Could you check a few things on this model? Use its own coordinates, in mm. Face numbers are marked on the shaded views. A direction names the side the tool comes from. Round coordinates to 2 decimals unless told otherwise and drop trailing zeros. Loops run counter-clockwise (first coordinate to the right, second up) from the corner with the lowest first, then second, coordinate; pieces in that order, holes last. Notation, with made-up numbers: (88, 72.5) - (121, 72.5) arc R13 cw to (121, 93.5) - close; hole circle Ø2 at (-5.75, -5). An arc over 180 degrees is marked (long way). Put each result on its own line as item: value. Start each with the question number.
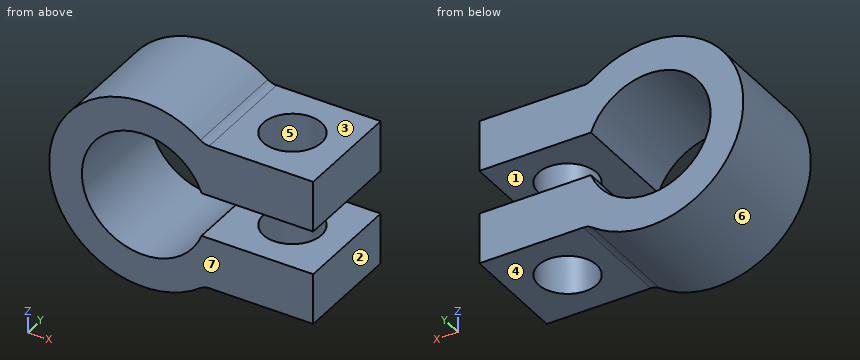
from build123d import *

# Parameters (mm, degrees)
SCHIZZO3_R           = 13
SCHIZZO3_R_2         = 8.5
ANELLO_DEPTH         = 15
AGGANCIOALTO_DEPTH   = 15
SCHIZZO5_W           = 23.306623863
SCHIZZO5_H           = 6
APERTURAANELLO_DEPTH = 31.61370144
SCHIZZO6_R           = 4
FOROPASSANTE_DEPTH   = 37.016644984
RACCORDOBASSO_R      = 2
RACCORDOALTO_R       = 2


with BuildPart() as part:
    # Schizzo3 → Anello (new body)
    with BuildSketch(Plane(origin=(0, 0, 0), x_dir=(1, 0, 0), z_dir=(0, 1, 0))):
        with Locations(Location((0, 0, 0), (0, 0, 270))):
            Circle(SCHIZZO3_R)
        with Locations(Location((0, 0, 0), (0, 0, 270))):
            Circle(SCHIZZO3_R_2, mode=Mode.SUBTRACT)
    extrude(amount=ANELLO_DEPTH)

    # Schizzo4 → AggancioAlto (add)
    with BuildSketch(Plane(origin=(0, 0, 0), x_dir=(1, 0, 0), z_dir=(0, 1, 0))):
        with BuildLine():
            Line((23.306623863, 3), (12.649110641, 3))
            ThreePointArc((12.649110641, 3), (11.046977059, 6.853050259), (8.306623863, 10))
            Line((8.306623863, 10), (23.306623863, 10))
            Line((23.306623863, 10), (23.306623863, 3))
        make_face()
    aggancioalto = extrude(amount=AGGANCIOALTO_DEPTH)

    # AggancioBasso: AggancioAlto across plane
    add(aggancioalto.mirror(Plane.XY))

    # Schizzo5 → AperturaAnello (cut, through all)
    with BuildSketch(Plane(origin=(0, 15, 0), x_dir=(1, 0, 0), z_dir=(0, 1, 0))):
        with Locations((11.653311932, 0)):
            Rectangle(SCHIZZO5_W, SCHIZZO5_H)
    extrude(amount=-APERTURAANELLO_DEPTH, mode=Mode.SUBTRACT)

    # Schizzo6 → ForoPassante (cut, through all)
    with BuildSketch(Plane.XY.offset(10)):
        with Locations((15.806623863, 7.5)):
            Circle(SCHIZZO6_R)
    extrude(amount=-FOROPASSANTE_DEPTH, mode=Mode.SUBTRACT)

    # RaccordoBasso
    raccordobasso_edges = [part.edges().sort_by_distance(p)[0] for p in [
        (8.306623863, 7.5, 10),
    ]]
    fillet(raccordobasso_edges, radius=RACCORDOBASSO_R)

    # RaccordoAlto
    raccordoalto_edges = [part.edges().sort_by_distance(p)[0] for p in [
        (8.306623863, 7.5, -10),
    ]]
    fillet(raccordoalto_edges, radius=RACCORDOALTO_R)


solid = part.part
Item 1: Suppose I cut it at C-C, the plane z = -7.75. List the corners of the cut face in (x, y) for me.
Item 2: Suppose I cut it at D-D, the plane x = 18.5. List the corners of the cut face in (y, z) for me.
Item 3: I need wall thicknesses on line 1 (Z direction, x = 21, y = 2.5); line 2 (Z direction, x = 0, y = 9.75); line 3 (X direction, y = 10, z = -7.75). Which ranges of each line are inside material? Lowest first, please. Write a range as from..to.
Item 4: Will these pins go through, and if not, where does the flat tip stop? P1, Ø3, axis at y = 5, z = 9.5, coming from the -X side; P2, Ø4.5, axis at x = 14.5, y = 9, coming from the +Z side; P3, Ø7.5, axis at x = 18.5, y = 9.5, coming from the -Z side.
Item 5: Suppose I cut it at B-B, the plane x = 0. List the corners of the cut face in (y, z) for me, then the cut area to 3 significant figures.
Item 6: On a 3-axis mill with a long thin cutter (end or side, diameter ignored), from which of +Z, -Z, +X, -X, +Y, -Y can I reach the whole of each face in a straight line? I mean the marked faces 1, 2, 3 and 4. Say none if no direction works.
Item 7: Suppose I cut it at A-A, the plane y = 7.5. List the corners of the cut face in (x, z) for me, then the cut area to 3 significant figures.
Item 8: Thinking about a two-plate mould opening in Y: for the marked faces 5, 6 and 7, which applies, released by +Y, released by -Y, zero draft, split by the parting line, or undercut?
Numbers:
1. outline: (-10.44, 0) - (-3.49, 0) - (-3.49, 15) - (-10.44, 15) - close; (3.49, 0) - (23.31, 0) - (23.31, 15) - (3.49, 15) - close; hole circle Ø8 at (15.81, 7.5)
2. outline: (0, -10) - (4.54, -10) - (4.54, -3) - (0, -3) - close; (0, 3) - (4.54, 3) - (4.54, 10) - (0, 10) - close; (10.46, -10) - (15, -10) - (15, -3) - (10.46, -3) - close; (10.46, 3) - (15, 3) - (15, 10) - (10.46, 10) - close
3. line 1: -10..-3, 3..10
3. line 2: -13..-8.5, 8.5..13
3. line 3: -10.44..-3.49, 3.49..12.68, 18.93..23.31
4. P1: x = -10.25
4. P2: z = 10
4. P3: z = -10
5. outline: (0, -13) - (15, -13) - (15, -8.5) - (0, -8.5) - close; (0, 8.5) - (15, 8.5) - (15, 13) - (0, 13) - close
5. area: 135 mm^2
6. face 1: +X, +Y, -Y
6. face 2: +Z, -Z, +X, +Y, -Y
6. face 3: +Z, +X, +Y, -Y
6. face 4: -Z, +X, +Y, -Y
7. outline: (7.8, -10.4) arc R2 cw to (9, -10) - (11.81, -10) - (11.81, -3) - (7.95, -3) arc R8.5 cw (long way) to (7.95, 3) - (11.81, 3) - (11.81, 10) - (9, 10) arc R2 cw to (7.8, 10.4) arc R13 ccw (long way) to start; (19.81, -10) - (23.31, -10) - (23.31, -3) - (19.81, -3) - close; (19.81, 3) - (23.31, 3) - (23.31, 10) - (19.81, 10) - close
7. area: 337 mm^2
8. face 5: undercut
8. face 6: zero draft
8. face 7: released by -Y
